Answer from the drawing. Dimensions are ordinates in mm from the lowest x, y and z of the part. A direction names the side the tool comes from. Coordinates: 2 decimals unless noted, no trailing zeros. Write each loop counter-clockwise with the first axis right and the second up, starting at its lowest first coordinate (ties: lowest second). Pieces come first, ordered by that corner, then holes.
1) Find the intervals of material crossed by line 1 (Y direction, x = 10.5, z = 1.9); line 2 (Y direction, x = 11.25, z = 4.7); line 3 (X direction, y = 9.5, z = 2.45), in increasing order.
2) The part is cut by section D-D (x = 13.75). Determine the outline of the cut face in (y, z), then the cut area to 3 significant figures.
3) Which of the six approach directions +Z, -Z, +X, -X, +Y, -Y give full straight-line access (tool end or side, diameter ignored) to the marked faces 5, 6 and 7?
4) Determine the mould class of the marked faces 1, 2, 3 and 4 for opening direction X: +X half, -X half, draft (parallel to the pull), parting line (faces both ways), or undercut.
5) The part is cut by section B-B (y = 11). Determine the outline of the cut face in (x, z), then the cut area to 3 significant figures.
6) The part is cut by section C-C (z = 4.2). Determine the outline of the cut face in (x, y), then the cut area to 3 significant figures.
7) The part is cut by section A-A (x = 4.5). Determine the outline of the cut face in (y, z).
8) Each of these flat-tipped pins is pushed along its axis until it touches: pin 1 Ø3 at (x, z) = (13.5, 5) entering from +Y; pin 2 Ø3 at (y, z) = (5.5, 1.5) entering from -X. Where does it stop, or does it pass through?
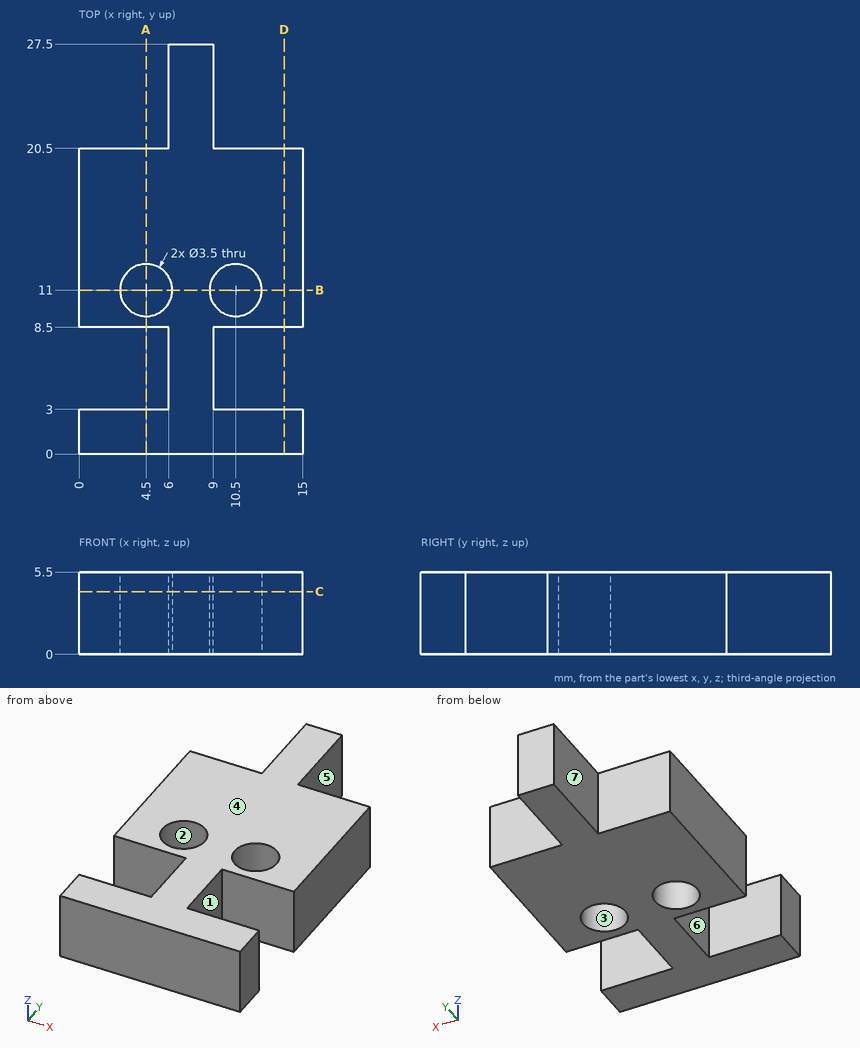
Reported:
1. line 1: y = 0 to 3, 8.5 to 9.25, 12.75 to 20.5
1. line 2: y = 0 to 3, 8.5 to 9.42, 12.58 to 20.5
1. line 3: x = 0 to 3.6, 5.4 to 9.6, 11.4 to 15
2. outline: (0, 0) - (3, 0) - (3, 5.5) - (0, 5.5) - close; (8.5, 0) - (20.5, 0) - (20.5, 5.5) - (8.5, 5.5) - close
2. area: 82.5 mm2
3. face 5: +Z, -Z, +X, +Y
3. face 6: +Z, -Z, -X
3. face 7: +Z, -Z, -X, +Y
4. face 1: +X half
4. face 2: undercut
4. face 3: undercut
4. face 4: draft
5. outline: (0, 0) - (2.75, 0) - (2.75, 5.5) - (0, 5.5) - close; (6.25, 0) - (8.75, 0) - (8.75, 5.5) - (6.25, 5.5) - close; (12.25, 0) - (15, 0) - (15, 5.5) - (12.25, 5.5) - close
5. area: 44.0 mm2
6. outline: (0, 0) - (15, 0) - (15, 3) - (9, 3) - (9, 8.5) - (15, 8.5) - (15, 20.5) - (9, 20.5) - (9, 27.5) - (6, 27.5) - (6, 20.5) - (0, 20.5) - (0, 8.5) - (6, 8.5) - (6, 3) - (0, 3) - close; hole circle Ø3.5 at (4.5, 11); hole circle Ø3.5 at (10.5, 11)
6. area: 243 mm2
7. outline: (0, 0) - (3, 0) - (3, 5.5) - (0, 5.5) - close; (8.5, 0) - (9.25, 0) - (9.25, 5.5) - (8.5, 5.5) - close; (12.75, 0) - (20.5, 0) - (20.5, 5.5) - (12.75, 5.5) - close
8. pin 1: stops at y = 20.5
8. pin 2: stops at x = 6
